Source: CAD feature listing. Evaluate the final solid. Frame: model axes, mm. Face numbers are marked on the shaded views. A direction names the side the tool comes from. Coordinates: 2 decimals unless noted, no trailing zeros. Write each loop counter-clockwise with the first axis right and the second up, starting at its lowest first coordinate (ties: lowest second). Pieces come first, ordered by that corner, then holes. Notation, with made-up numbers: M 28,8.25 L 67,8.25 A18 cw 67,28.25 Z; hole C 79,56 d6. An arc over 180 degrees is marked long. Write item = value, one per line. Start each with the question number.
1. Access query for the marked faces 1 and 2. Directions: +Z, -Z, +X, -X, +Y, -Y. A direction counts if a zero-diameter tool reaches every point of the face in a straight line with its end or side. Return the directions, or none.
2. Section query C-C (z = 13). Output: boundary loops of the cut face in (x, y) (3 decimals).
3. Pull-direction query (X, two-part tool) for the marked faces 3, 4, 5 and 6; classes: pulls with the +X half, pulls with the -X half, needs draft (parallel to the pull), parting line crosses it, or undercut.
4. Section query D-D (x = -27). Output: boundary loops of the cut face in (y, z).
5. Line query: line 1 along Y through (x, z) = (-6.5, 0.4); line 2 along Y through (x, z) = (-1.8, 15.5); line 3 along X through (y, z) = (-30.2, 12.5). Output: solid intervals per line, ascending.
6. Section query A-A (x = -35). Output: boundary loops of the cut face in (y, z) (3 decimals), then the cut area to 3 significant figures.
7. Section query B-B (y = -7). Output: boundary loops of the cut face in (x, z) (3 decimals), then the cut area to 3 significant figures.
8. Pin query (flat end, axial travel): pin 1 Ø8 at (x, y) = (-22, -15) entering from +Z; pin 2 Ø5.5 at (x, y) = (-39.5, -7) entering from -Z; pin 3 Ø2.5 at (x, y) = (-1.8, -30.2) entering from -Z. Return the tip coordinate at first contact, or that it passes through.
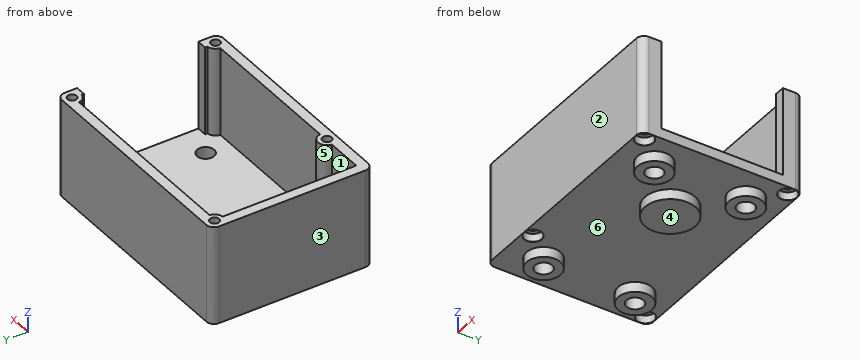
```python
from build123d import *

# Parameters (mm, degrees)
SKETCH2_W                       = 46
SKETCH2_H                       = 32
BOSS_EXTRUDE1_DEPTH             = 19.5
SHELL1_T                        = -2
CBORE_FOR_M3_SBHCS1_AT_2_COUNT  = 2
CBORE_FOR_M3_SBHCS1_AT_2_PITCH  = 18.114862856
CBORE_FOR_M3_SBHCS1_AT_3_COUNT  = 2
CBORE_FOR_M3_SBHCS1_AT_3_PITCH  = 37.645029636
CBORE_FOR_M3_SBHCS1_AT_4_COUNT  = 2
CBORE_FOR_M3_SBHCS1_AT_4_PITCH  = 33
SKETCH8_R                       = 3.35
SKETCH8_R_2                     = 1.7
BOSS_EXTRUDE2_DEPTH             = 3.63
SKETCH9_R                       = 5
BOSS_EXTRUDE3_DEPTH             = 2
SKETCH10_W                      = 17.5
SKETCH10_H                      = 24
CUT_EXTRUDE1_DEPTH              = 2
CBORE_FOR_M1_6_SHCS1_AT_2_COUNT = 2
CBORE_FOR_M1_6_SHCS1_AT_2_PITCH = 42.4
CBORE_FOR_M1_6_SHCS1_AT_3_COUNT = 2
CBORE_FOR_M1_6_SHCS1_AT_3_PITCH = 43.689815747
CBORE_FOR_M1_6_SHCS1_AT_4_COUNT = 2
CBORE_FOR_M1_6_SHCS1_AT_4_PITCH = 28.4
SKETCH14_R                      = 1.75
SKETCH14_R_2                    = 0.9
SKETCH14_R_3                    = 1.775
BOSS_EXTRUDE4_DEPTH             = 17.9
FILLET1_R                       = 1.5


with BuildPart() as part:
    # Sketch2 → Boss-Extrude1 (new body)
    with BuildSketch(Plane.XY):
        with Locations((-23, -16)):
            Rectangle(SKETCH2_W, SKETCH2_H)
    extrude(amount=BOSS_EXTRUDE1_DEPTH)

    # Shell1
    shell1_openings = [part.faces().sort_by_distance(p)[0] for p in [
        (-23, -16, 19.5),
    ]]
    offset(amount=SHELL1_T, openings=shell1_openings, kind=Kind.INTERSECTION)

    # Sketch5 → CBORE for M3 SBHCS1 (revolve, cut)
    with BuildSketch(Plane(origin=(-6.5, -7, 0), x_dir=(0, 1, 0), z_dir=(1, 0, 0))):
        Polygon((0, 0), (0, 3.021463052), (1.7, 2), (1.7, 1.65), (3.35, 1.65), (3.35, 0.025), (3.375, 0), align=None)
    cbore_for_m3_sbhcs1 = revolve(axis=Axis((-6.5, -7, -6.35), (0, 0, 1)), mode=Mode.SUBTRACT)

    # CBORE for M3 SBHCS1 at 2: CBORE for M3 SBHCS1 ×2
    with Locations(*[(0, -i * CBORE_FOR_M3_SBHCS1_AT_2_PITCH, 0) for i in range(1, CBORE_FOR_M3_SBHCS1_AT_2_COUNT)]):
        add(cbore_for_m3_sbhcs1, mode=Mode.SUBTRACT)

    # CBORE for M3 SBHCS1 at 3: CBORE for M3 SBHCS1 ×2
    with Locations(*[Vector(-0.8766097495224606, -0.4812019815443084, 0) * (i * CBORE_FOR_M3_SBHCS1_AT_3_PITCH) for i in range(1, CBORE_FOR_M3_SBHCS1_AT_3_COUNT)]):
        add(cbore_for_m3_sbhcs1, mode=Mode.SUBTRACT)

    # CBORE for M3 SBHCS1 at 4: CBORE for M3 SBHCS1 ×2
    with Locations(*[(-i * CBORE_FOR_M3_SBHCS1_AT_4_PITCH, 0, 0) for i in range(1, CBORE_FOR_M3_SBHCS1_AT_4_COUNT)]):
        add(cbore_for_m3_sbhcs1, mode=Mode.SUBTRACT)

    # Sketch8 → Boss-Extrude2 (add)
    # profile 1 of 4: a face of its own
    with BuildSketch(Plane(origin=(0, 0, 1.65), x_dir=(-1, 0, 0), z_dir=(0, 0, -1))):
        with Locations((6.5, -25.114862856)):
            Circle(SKETCH8_R)
        with Locations((6.5, -25.114862856)):
            Circle(SKETCH8_R_2, mode=Mode.SUBTRACT)
    # profile 2 of 4: a face of its own
    with BuildSketch(Plane(origin=(0, 0, 1.65), x_dir=(-1, 0, 0), z_dir=(0, 0, -1))):
        with Locations((39.5, -25.114862856)):
            Circle(SKETCH8_R)
        with Locations((39.5, -25.114862856)):
            Circle(SKETCH8_R_2, mode=Mode.SUBTRACT)
    # profile 3 of 4: a face of its own
    with BuildSketch(Plane(origin=(0, 0, 1.65), x_dir=(-1, 0, 0), z_dir=(0, 0, -1))):
        with Locations((39.5, -7)):
            Circle(SKETCH8_R)
        with Locations((39.5, -7)):
            Circle(SKETCH8_R_2, mode=Mode.SUBTRACT)
    # profile 4 of 4: a face of its own
    with BuildSketch(Plane(origin=(0, 0, 1.65), x_dir=(-1, 0, 0), z_dir=(0, 0, -1))):
        with Locations((6.5, -7)):
            Circle(SKETCH8_R)
        with Locations((6.5, -7)):
            Circle(SKETCH8_R_2, mode=Mode.SUBTRACT)
    extrude(amount=BOSS_EXTRUDE2_DEPTH)

    # Sketch9 → Boss-Extrude3 (add)
    with BuildSketch(Plane(origin=(0, 0, 0), x_dir=(-1, 0, 0), z_dir=(0, 0, -1))):
        with Locations((15.5, -16)):
            Circle(SKETCH9_R)
    extrude(amount=BOSS_EXTRUDE3_DEPTH)

    # Sketch10 → Cut-Extrude1 (cut)
    with BuildSketch(Plane(origin=(0, 0, 0), x_dir=(0, 0, -1), z_dir=(1, 0, 0))):
        with Locations((-10.75, -16)):
            Rectangle(SKETCH10_W, SKETCH10_H)
    extrude(amount=-CUT_EXTRUDE1_DEPTH, mode=Mode.SUBTRACT)

    # Sketch13 → CBORE for M1.6 SHCS1 (revolve, cut)
    with BuildSketch(Plane(origin=(-1.8, -1.8, 0), x_dir=(0, 1, 0), z_dir=(1, 0, 0))):
        Polygon((0, 0), (0, 19.5), (0.9, 19.5), (0.9, 1.6), (1.75, 1.6), (1.75, 0.025), (1.775, 0), align=None)
    cbore_for_m1_6_shcs1 = revolve(axis=Axis((-1.8, -1.8, -6.35), (0, 0, 1)), mode=Mode.SUBTRACT)

    # CBORE for M1.6 SHCS1 at 2: CBORE for M1.6 SHCS1 ×2
    with Locations(*[(-i * CBORE_FOR_M1_6_SHCS1_AT_2_PITCH, 0, 0) for i in range(1, CBORE_FOR_M1_6_SHCS1_AT_2_COUNT)]):
        add(cbore_for_m1_6_shcs1, mode=Mode.SUBTRACT)

    # CBORE for M1.6 SHCS1 at 3: CBORE for M1.6 SHCS1 ×2
    with Locations(*[Vector(-0.759902495179072, -0.6500370741893268, 0) * (i * CBORE_FOR_M1_6_SHCS1_AT_3_PITCH) for i in range(1, CBORE_FOR_M1_6_SHCS1_AT_3_COUNT)]):
        add(cbore_for_m1_6_shcs1, mode=Mode.SUBTRACT)

    # CBORE for M1.6 SHCS1 at 4: CBORE for M1.6 SHCS1 ×2
    with Locations(*[(0, -i * CBORE_FOR_M1_6_SHCS1_AT_4_PITCH, 0) for i in range(1, CBORE_FOR_M1_6_SHCS1_AT_4_COUNT)]):
        add(cbore_for_m1_6_shcs1, mode=Mode.SUBTRACT)

    # Sketch14 → Boss-Extrude4 (add)
    # profile 1 of 4: a face of its own
    with BuildSketch(Plane(origin=(0, 0, 1.6), x_dir=(-1, 0, 0), z_dir=(0, 0, -1))):
        with Locations((1.8, -1.8)):
            Circle(SKETCH14_R)
        with Locations((1.8, -1.8)):
            Circle(SKETCH14_R_2, mode=Mode.SUBTRACT)
    # profile 2 of 4: a face of its own
    with BuildSketch(Plane(origin=(0, 0, 1.6), x_dir=(-1, 0, 0), z_dir=(0, 0, -1))):
        with Locations((44.2, -1.8)):
            Circle(SKETCH14_R_3)
        with Locations((44.2, -1.8)):
            Circle(SKETCH14_R_2, mode=Mode.SUBTRACT)
    # profile 3 of 4: a face of its own
    with BuildSketch(Plane(origin=(0, 0, 1.6), x_dir=(-1, 0, 0), z_dir=(0, 0, -1))):
        with Locations((35, -30.2)):
            Circle(SKETCH14_R_3)
        with Locations((35, -30.2)):
            Circle(SKETCH14_R_2, mode=Mode.SUBTRACT)
    # profile 4 of 4: a face of its own
    with BuildSketch(Plane(origin=(0, 0, 1.6), x_dir=(-1, 0, 0), z_dir=(0, 0, -1))):
        with Locations((1.8, -30.2)):
            Circle(SKETCH14_R)
        with Locations((1.8, -30.2)):
            Circle(SKETCH14_R_2, mode=Mode.SUBTRACT)
    extrude(amount=-BOSS_EXTRUDE4_DEPTH)

    # Fillet1
    fillet1_edges = [part.edges().sort_by_distance(p)[0] for p in [
        (0, -32, 9.75),
        (-46, -32, 9.75),
        (-46, 0, 9.75),
        (0, 0, 9.75),
    ]]
    fillet(fillet1_edges, radius=FILLET1_R)


solid = part.part
```
Results are:
q1.face_1 = +Z
q1.face_2 = +Z, -Z, +X, -X, -Y
q2.outline = M -46,-30.5 A1.5 ccw -44.5,-32 L -1.5,-32 A1.5 ccw 0,-30.5 L 0,-28 L -2,-28 L -2,-28.461 A1.75 ccw -3.539,-30 L -33.236,-30 A1.775 ccw -36.764,-30 L -44,-30 L -44,-3.564 A1.775 ccw -42.436,-2 L -3.539,-2 A1.75 ccw -2,-3.539 L -2,-4 L 0,-4 L 0,-1.5 A1.5 ccw -1.5,0 L -44.5,0 A1.5 ccw -46,-1.5 Z; hole C -44.2,-1.8 d1.8; hole C -35,-30.2 d1.8; hole C -1.8,-30.2 d1.8; hole C -1.8,-1.8 d1.8
q3.face_3 = pulls with the -X half
q3.face_4 = needs draft
q3.face_5 = undercut
q3.face_6 = undercut
q4.outline = M -32,0 L 0,0 L 0,19.5 L -2,19.5 L -2,2 L -30,2 L -30,19.5 L -32,19.5 Z
q5.line_1 = -32 to -26.81, -23.41 to -8.7, -5.3 to 0
q5.line_2 = -32 to -31.1, -29.3 to -28, -4 to -2.7, -0.9 to 0
q5.line_3 = -46 to -35.9, -34.1 to -2.7, -0.9 to 0
q6.outline = M -32,0 L -31.975,0 L -31.95,0.025 L -31.95,1.6 L -31.1,1.6 L -31.1,19.5 L -32,19.5 Z; M -29.3,1.6 L -28.45,1.6 L -28.45,0.025 L -28.425,0 L 0,0 L 0,19.5 L -2,19.5 L -2,2 L -28.425,2 L -28.425,19.5 L -29.3,19.5 Z
q6.area = 124 mm^2
q7.outline = M -46,0 L -42.875,0 L -42.85,0.025 L -42.85,-1.98 L -41.2,-1.98 L -41.2,2 L -44,2 L -44,19.5 L -46,19.5 Z; M -37.8,-1.98 L -36.15,-1.98 L -36.15,0.025 L -36.125,0 L -9.875,0 L -9.85,0.025 L -9.85,-1.98 L -8.2,-1.98 L -8.2,2 L -37.8,2 Z; M -4.8,-1.98 L -3.15,-1.98 L -3.15,0.025 L -3.125,0 L 0,0 L 0,2 L -4.8,2 Z
q7.area = 126 mm^2
q8.pin_1 = 2
q8.pin_2 = -1.98
q8.pin_3 = 1.6
